Verification items for the finished model (mm, model axes). Face numbers are marked on the shaded views. A direction names the side the tool comes from. Give positions to 0.01 mm unless a question says otherwise; leave off trailing zeros. Order: outer loops, then holes, each group sorted by start corner. A loop starts at its lowest first (then second) coordinate and runs counter-clockwise, first axis right, second up. Notation, with made-up numbers: (65, 86) -> (89, 86) arc R9 ccw to (89, 94) -> close; hole circle Ø3 at (32.5, 40.5). An arc over 180 degrees is marked (long way). One line per question, with ' | ' between items. Start each with the question number.
Q1. Access from +Z, -Z, +X, -X, +Y, -Y to the whole of each face (thin tool, end or side, straight path). Record for the marked faces 4, 5, 6 and 7.
Q2. Section check D-D on y = 4. Record the cut outline in (x, z).
Q3. Section check B-B on y = -0.1. Record the cut outline in (x, z), plus the area to 3 significant figures.
Q4. Section check A-A on x = 16. Record the cut outline in (y, z), plus the area to 3 significant figures.
Q5. Material ranges on probe 1 along X at (y, z) = (-0.1, 1.45); probe 2 along X at (y, z) = (-1, 2.5); probe 3 along X at (y, z) = (4.5, 0), recorded low to high. Write a range as [from, to].
Q6. Go/stop test with flat-tipped pins: pin 1 (3 mm diameter, centred on x = 16, y = -0.1, fed in from +Z); pin 2 (3 mm diameter, centred on y = 4.5, z = 0, fed in from -X); pin 3 (7.5 mm diameter, centred on x = 4, y = 0.5, fed in from -Z). Record where each tip stops, or that it passes through.
Q7. Mould release check, pull along X, two halves, no side actions. Record for the marked faces 1, 2 and 3: released by +X, released by -X, zero draft, split by the parting line, or undercut.
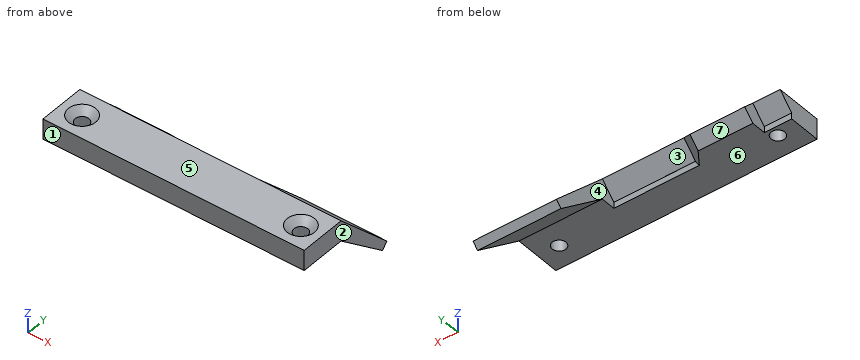
Autodesk Inventor part; units mm, degrees
ref_plane "YZ Plane" through (0, 0, 0) normal (1, 0, 0) x (0, 1, 0)
ref_plane "XZ Plane" through (0, 0, 0) normal (0, 1, 0) x (-1, 0, 0)
ref_plane "XY Plane" through (0, 0, 0) normal (0, 0, 1) x (1, 0, 0)
sketch "Sketch1" plane through (0, 0, 0) normal (0, 0, 1) x (1, 0, 0)
  line L0 (-19.1, 3.4) -> (19.1, 3.4)
  line L1 (19.1, 3.4) -> (19.1, -3.4)
  line L2 (19.1, -3.4) -> (-19.1, -3.4)
  line L3 (-19.1, -3.4) -> (-19.1, 3.4)
  point P0 (0, 0)
  dimension "d0" = 38.2
  dimension "d1" = 6.8
  dimension "d2" = 19.1
  dimension "d3" = 3.4
extrude "Extrusion1" add sketch "Sketch1" along normal blind 3
sketch "Sketch2" plane through (0, 0, 3) normal (0, 0, 1) x (1, 0, 0)
  line L0 (19.1, 3.4) -> (-19.1, 3.4)
  line L1 (-19.1, 3.4) -> (-19.1, -3.4)
  line L2 (19.1, -3.4) -> (19.1, 3.4)
  point P0 (0, 0)
  point P1 (-16, -0.1)
  point P2 (16, -0.1)
  point P3 (-16, -0.1)
  dimension "d6" = 3.5
  dimension "d7" = 3.5
  dimension "d8" = 32
  dimension "d9" = 3.1
  dimension "d10" = 3.1
hole "Hole1" at (-16, -0.1, 3) at (16, -0.1, 3) direction (0, 0, -1) diameter 2 depth 4 tip angle 118 countersink diameter 4 countersink angle 90
sketch "Sketch3" plane through (19.1, -3.4, 0) normal (1, 0, 0) x (0, 0, -1)
  line L0 (-3, 6.8) -> (-3, 0)
  line L1 (-3, 6.8) -> (5.4853, 15.2853)
  line L2 (-3, 6.8) -> (9, 6.8) construction
  line L3 (5.4853, 15.2853) -> (6.3338, 14.4368)
  line L4 (0, 0) -> (0, 6.8)
  line L5 (6.3338, 14.4368) -> (0, 6.8)
  line L6 (0, 6.8) -> (-3, 6.8)
  point P0 (0, 3.4)
  dimension "d18" = 12
  dimension "d19" = 45
  dimension "d20" = 1.2
extrude "Extrusion2" add sketch "Sketch3" against normal blind 38.2
sketch "Sketch4" plane through (-19.1, 11.8853, -5.4853) normal (0, 0.7071, 0.7071) x (1, 0, 0)
  line L0 (0, -12) -> (0, 0)
  line L1 (38.2, -12) -> (0, -12)
  line L2 (0, 0) -> (4, 0)
  line L3 (4, 0) -> (4, -12)
  line L4 (4, -12) -> (0, -12)
  line L5 (0, -12) -> (0, 0)
  line L6 (38.2, 0) -> (0, 0)
  line L7 (38.2, -9.8787) -> (0, -9.8787)
  line L8 (4, 0) -> (14, 0)
  line L9 (14, 0) -> (14, -9.8787)
  line L10 (14, -9.8787) -> (4, -9.8787)
  line L11 (4, -9.8787) -> (4, 0)
  line L12 (14, 0) -> (26, 0)
  line L13 (26, 0) -> (26, -12)
  line L14 (26, -12) -> (14, -12)
  line L15 (14, -12) -> (14, 0)
  point P0 (19.1, -12.2828)
  point P1 (4, -9.8787)
  point P2 (14, -9.8787)
  dimension "d23" = 4
  dimension "d24" = 4
  dimension "d25" = 14
  dimension "d26" = 26
extrude "Extrusion3" cut sketch "Sketch4" against normal blind 3 contours L0 L7 L3 L1 | L0 L2 L3 L7 | L3 L6 L9 L7 | L15 L7 L13 L1 | L9 L6 L13 L7
sketch "Sketch5" plane through (0, 0, 0) normal (0, 0, -1) x (-1, 0, 0)
  line L0 (5.1, 2.1574) -> (-6.9, 2.1574)
  line L1 (-6.9, 1.2787) -> (5.1, 1.2787)
  line L2 (-6.9, 2.1574) -> (5.1, 2.1574)
  line L3 (5.1, 2.1574) -> (5.1, 1.2787)
  line L4 (5.1, 1.2787) -> (-6.9, 1.2787)
  line L5 (-6.9, 1.2787) -> (-6.9, 2.1574)
  line L6 (15.1, 2.1574) -> (15.1, 1.2787)
  line L7 (15.1, 1.2787) -> (19.1, 1.2787)
  line L8 (15.1, 2.1574) -> (19.1, 2.1574)
  line L9 (19.1, 2.1574) -> (19.1, 1.2787)
  line L10 (19.1, 1.2787) -> (15.1, 1.2787)
  line L11 (15.1, 1.2787) -> (15.1, 2.1574)
  point P0 (0, 0)
extrude "Extrusion4" cut sketch "Sketch5" against normal blind 0.88
chamfer "Chamfer1" distance 2 angle 45 1 edges at (-5.1, 4.15, 0.75)
properties part number "display_mount"
Filled in:
1) face 4: -Z, +Y | face 5: +Z, +X, -X, +Y, -Y | face 6: -Z, +X, -X, -Y | face 7: -Z, -X, +Y
2) outline: (-15.1, 0.6) -> (-7.1, 0.6) -> (-5.83, 2.4) -> (-15.1, 2.4) -> close; (6.9, -0.5) -> (19.1, -0.5) -> (19.1, 2.4) -> (6.9, 2.4) -> close
3) outline: (-19.1, 0) -> (-17, 0) -> (-17, 2) -> (-18, 3) -> (-19.1, 3) -> close; (-15, 0) -> (15, 0) -> (15, 2) -> (14, 3) -> (-14, 3) -> (-15, 2) -> close; (17, 0) -> (19.1, 0) -> (19.1, 3) -> (18, 3) -> (17, 2) -> close | area: 101 mm²
4) outline: (-3.4, 0) -> (-1.1, 0) -> (-1.1, 2) -> (-2.1, 3) -> (-3.4, 3) -> close; (0.9, 0) -> (3.4, 0) -> (11.04, -6.33) -> (11.89, -5.49) -> (3.4, 3) -> (1.9, 3) -> (0.9, 2) -> close | area: 32.1 mm²
5) probe 1: [-19.1, -17], [-15, 15], [17, 19.1] | probe 2: [-19.1, -17.2], [-14.8, 14.8], [17.2, 19.1] | probe 3: [6.9, 19.1]
6) pin 1: z = 2.5 | pin 2: x = -15.1 | pin 3: z = 0
7) face 1: zero draft | face 2: released by +X | face 3: undercut
